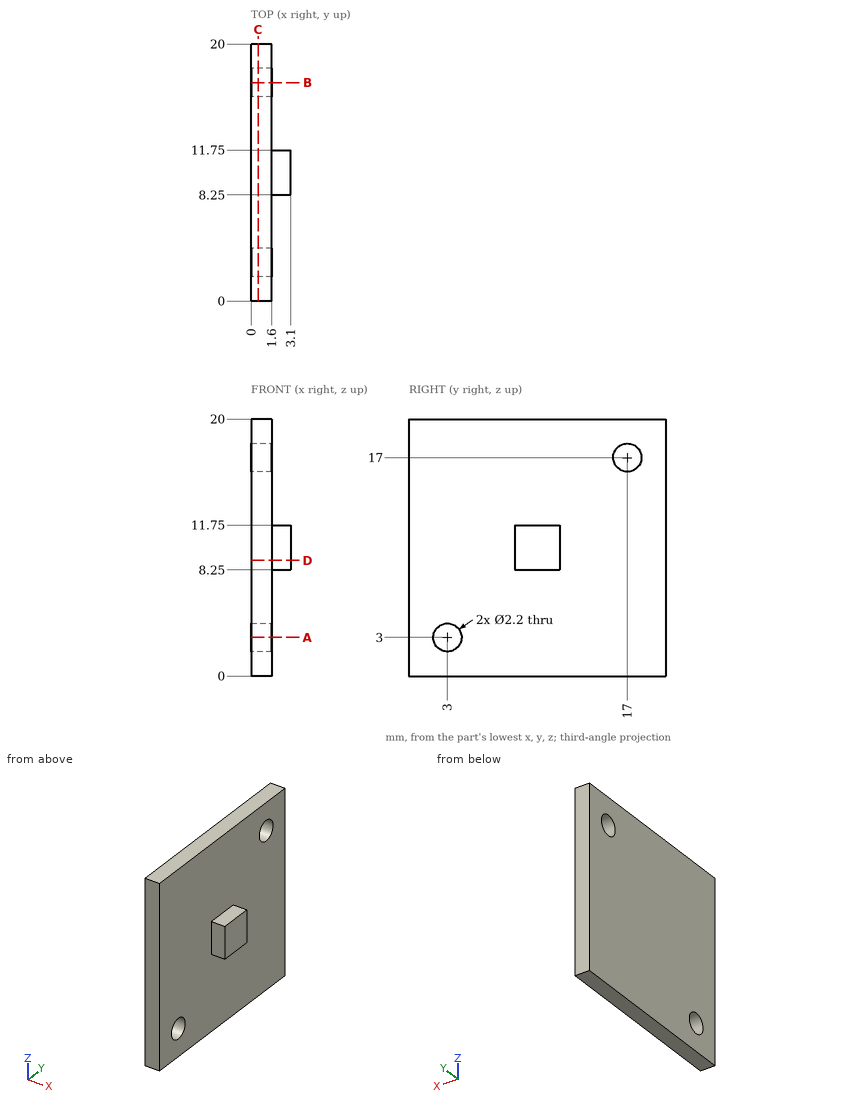
The figure shows three views and two pictorial views of one solid part (mm, origin at its lowest corner). Answer the questions. Coordinates: 2 decimals unless noted, no trailing zeros. Write each loop counter-clockwise with the first axis right and the second up, starting at its lowest first coordinate (ties: lowest second). Pieces come first, ordered by that corner, then holes. Notation, with made-up numbers: (47.5, 57.25) -> (74.5, 57.25) arc R26 ccw to (74.5, 89.25) -> close; hole circle Ø7 at (28.25, 81). An arc over 180 degrees is marked (long way). Answer as a JSON object with one key per item and string values.
Q1. The part is cut by section A-A on z = 3. Give the vertices of the cut face in (x, y), then the cut area to 3 significant figures.
The answers:
{"outline": "(0, 0) -> (1.6, 0) -> (1.6, 1.9) -> (0, 1.9) -> close; (0, 4.1) -> (1.6, 4.1) -> (1.6, 20) -> (0, 20) -> close", "area": "28.5 mm2"}
Q2. The part is cut by section D-D on z = 9. Give the vertices of the cut face in (x, y).
The answers:
{"outline": "(0, 0) -> (1.6, 0) -> (1.6, 8.25) -> (3.1, 8.25) -> (3.1, 11.75) -> (1.6, 11.75) -> (1.6, 20) -> (0, 20) -> close"}
Q3. Consider line 1 (Y direction, x = 1.05, z = 3); line 2 (Y direction, x = 0.45, z = 17); line 3 (X direction, y = 11, z = 16). Determine where each line is inside the solid, lowest interval first. Write a range as [from, to].
The answers:
{"line 1": "y = [0, 1.9], [4.1, 20]", "line 2": "y = [0, 15.9], [18.1, 20]", "line 3": "x = [0, 1.6]"}
Q4. The part is cut by section C-C on x = 0.55. Give the vertices of the cut face in (y, z).
The answers:
{"outline": "(0, 0) -> (20, 0) -> (20, 20) -> (0, 20) -> close; hole circle Ø2.2 at (3, 3); hole circle Ø2.2 at (17, 17)"}
Q5. Flat-ended cylindrical pins translate along their axes: pin 1 Ø1.5 at (x, y) = (1.5, 8) entering from -Z; pin 2 Ø1.6 at (x, y) = (2.5, 10) entering from -Z; pin 3 Ø1 at (y, z) = (7.5, 16.5) entering from +X; pin 4 Ø1.2 at (x, z) = (2.5, 9.5) entering from -Y. Find the tip coordinate at first contact, or state that the pin passes through.
The answers:
{"pin 1": "stops at z = 0", "pin 2": "stops at z = 8.25", "pin 3": "stops at x = 1.6", "pin 4": "stops at y = 8.25"}
Q6. The part is cut by section B-B on y = 17. Give the vertices of the cut face in (x, z).
The answers:
{"outline": "(0, 0) -> (1.6, 0) -> (1.6, 15.9) -> (0, 15.9) -> close; (0, 18.1) -> (1.6, 18.1) -> (1.6, 20) -> (0, 20) -> close"}
